Input: part model. Units: mm. Frame: model coordinates. Give positions to 0.01 mm unless a question says otherwise; leave off trailing zeros. Loops run counter-clockwise (first coordinate to the right, second up) from the corner with the lowest first, then second, coordinate; pieces in that order, holes last. Notation, with made-up numbers: M 27,36 L 45,36 A21 cw 45,58 Z; hole C -31.5,-35.5 d4. An arc over 180 degrees is marked long. One line per item, written item: value. Start each with the question number.
(1) Pin query (flat end, axial travel): P1, Ø0.6, axis at y = 20, z = 1, coming from the -X side; P2, Ø1, axis at y = 26, z = 0.5, coming from the +X side; P3, Ø1, axis at x = 9, z = 1, coming from the +Y side. Return the tip coordinate at first contact, or that it passes through.
(2) Ray query, line 1 along Y through (x, z) = (0, 0.75); line 2 along Y through (x, z) = (53, 1.7); line 3 along X through (y, z) = (23, 0.8). Return the intervals inside material, ascending. Write a range as from..to.
(3) Section D-D on x = 15. Output: boundary loops of the cut face in (y, z).
(4) Section C-C on z = 0.65. State how many separate pieces and enclosed holes the cut face has, plus the area to 3 significant figures.
(5) Section A-A on y = 0. Output: boundary loops of the cut face in (x, z).
(6) Section B-B on x = 35. Output: boundary loops of the cut face in (y, z), plus the area to 3 significant figures.
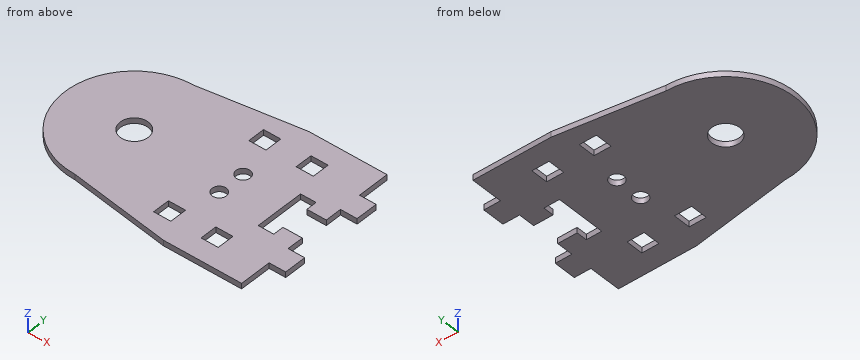
```python
from build123d import *

# Parameters (mm, degrees)
SKETCH_1_R      = 5.05
SKETCH_1_R_2    = 2.55
SKETCH_1_W      = 6.2
SKETCH_1_H      = 6.2
EXTRUDE_1_DEPTH = 2


with BuildPart() as part:
    # 草图1 → 凸台-拉伸1 (new body)
    with BuildSketch(Plane.XY):
        with BuildLine():
            Line((0, -25), (36.822908512, -30.548036369))
            Line((36.822908512, -30.548036369), (65, -30.548036369))
            Line((65, -30.548036369), (65, -19))
            Line((65, -19), (71, -19))
            Line((71, -19), (71, -11))
            Line((71, -11), (65, -11))
            Line((65, -11), (65, -5.05))
            Line((65, -5.05), (58, -5.05))
            Line((58, -5.05), (58, -8.9))
            Line((58, -8.9), (52.4, -8.9))
            Line((52.4, -8.9), (52.4, -5.15))
            Line((52.4, -5.15), (52.4, 5.15))
            Line((52.4, 5.15), (52.4, 8.9))
            Line((52.4, 8.9), (58, 8.9))
            Line((58, 8.9), (58, 5.05))
            Line((58, 5.05), (65, 5.05))
            Line((65, 5.05), (65, 11))
            Line((65, 11), (71, 11))
            Line((71, 11), (71, 19))
            Line((71, 19), (65, 19))
            Line((65, 19), (65, 30.548036369))
            Line((65, 30.548036369), (36.822908512, 30.548036369))
            Line((36.822908512, 30.548036369), (0, 25))
            ThreePointArc((0, 25), (-25, 0), (0, -25))
        make_face()
        Circle(SKETCH_1_R, mode=Mode.SUBTRACT)
        with Locations((35, 5)):
            Circle(SKETCH_1_R_2, mode=Mode.SUBTRACT)
        with Locations(Location((35, -5, 0), (0, 0, 180))):
            Circle(SKETCH_1_R_2, mode=Mode.SUBTRACT)
        with Locations((47.05, -20)):
            Rectangle(SKETCH_1_W, SKETCH_1_H, mode=Mode.SUBTRACT)
        with Locations((29.95, -20)):
            Rectangle(SKETCH_1_W, SKETCH_1_H, mode=Mode.SUBTRACT)
        with Locations((29.95, 20)):
            Rectangle(SKETCH_1_W, SKETCH_1_H, mode=Mode.SUBTRACT)
        with Locations((47.05, 20)):
            Rectangle(SKETCH_1_W, SKETCH_1_H, mode=Mode.SUBTRACT)
    extrude(amount=EXTRUDE_1_DEPTH)


solid = part.part
```
Output values:
1. P1: stops at x = -15.39
1. P2: stops at x = 65
1. P3: stops at y = 26.43
2. line 1: y = -25..-5.05, 5.05..25
2. line 2: y = -30.55..-8.9, 8.9..30.55
2. line 3: x = -9.8..26.85, 33.05..43.95, 50.15..65
3. outline: M -27.26,0 L 27.26,0 L 27.26,2 L -27.26,2 Z
4. separate pieces: 1
4. enclosed holes: 7
4. area: 4,400 mm²
5. outline: M -25,0 L -5.05,0 L -5.05,2 L -25,2 Z; M 5.05,0 L 52.4,0 L 52.4,2 L 5.05,2 Z
6. outline: M -30.27,0 L -7.55,0 L -7.55,2 L -30.27,2 Z; M -2.45,0 L 2.45,0 L 2.45,2 L -2.45,2 Z; M 7.55,0 L 30.27,0 L 30.27,2 L 7.55,2 Z
6. area: 101 mm²
